```python
from build123d import *

# Parameters (mm, degrees)
SKETCH_1_W          = 10
SKETCH_1_H          = 10
SKETCH_1_W_2        = 8
SKETCH_1_H_2        = 8
EXTRUDE_1_DEPTH     = 20
SKETCH_3_R          = 1.6
CUT_EXTRUDE_1_DEPTH = 23.912878475
SKETCH_4_R          = 1.6
CUT_EXTRUDE_2_DEPTH = 23.912878475


with BuildPart() as part:
    # ｽｹｯﾁ1 → ﾎﾞｽ - 押し出し1 (new body)
    with BuildSketch(Plane.XY):
        Rectangle(SKETCH_1_W, SKETCH_1_H)
        Rectangle(SKETCH_1_W_2, SKETCH_1_H_2, mode=Mode.SUBTRACT)
    extrude(amount=EXTRUDE_1_DEPTH)

    # ｽｹｯﾁ3 → ｶｯﾄ - 押し出し1 (cut, through all)
    with BuildSketch(Plane(origin=(0, 5, 0), x_dir=(1, 0, 0), z_dir=(0, 1, 0))):
        with Locations(Location((0, -5, 0), (0, 0, 270))):
            Circle(SKETCH_3_R)
    extrude(amount=-CUT_EXTRUDE_1_DEPTH, mode=Mode.SUBTRACT)

    # ｽｹｯﾁ4 → ｶｯﾄ - 押し出し2 (cut, through all)
    with BuildSketch(Plane.ZY.offset(5)):
        with Locations(Location((15, 0, 0), (0, 0, 270))):
            Circle(SKETCH_4_R)
    extrude(amount=-CUT_EXTRUDE_2_DEPTH, mode=Mode.SUBTRACT)


solid = part.part
```
The model under review builds one solid part; all positions refer to its coordinate system, in mm. A direction names the side the tool comes from. Round coordinates to 2 decimals unless told otherwise and drop trailing zeros. Loops run counter-clockwise (first coordinate to the right, second up) from the corner with the lowest first, then second, coordinate; pieces in that order, holes last. Notation, with made-up numbers: (-17.75, 76.25) -> (8.25, 76.25) arc R19 ccw to (8.25, 104.25) -> close; hole circle Ø9 at (22.25, 17). An arc over 180 degrees is marked (long way). Answer as a JSON object with one key per item and string values. Group by question number.
1) We need section A-A on x = -3.75. Write out the cut boundary in (y, z), then the cut area to 3 significant figures.
2) For line 1 (X direction, y = 0, z = 2.25); line 2 (X direction, y = 4.25, z = 5.5), list the stretches that pass through material, from the lowest coordinate up. Write a range as [from, to].
3) Mouldability with a two-part tool opening along Y and no side actions: class faces 3 (the face through (5, 0, 10)), 4 (the face through (0, -5, 10)), 5 (the face through (0, 4, 10)) as released by +Y, released by -Y, zero draft, split by the parting line, or undercut.
4) We need section B-B on z = 9.25. Write out the cut boundary in (x, y).
5) We need section C-C on y = 0. Write out the cut boundary in (x, z), then the cut area to 3 significant figures.
6) For pin 1 Ø3.5 at (x, z) = (0, 5) entering from +Y, flat-tipped, find the tip position at first contact; note if it passes through.
7) For faces 1 (the face through (-4.5, 0.1, 0)), 2 (the face through (-4, 0, 10)), list the 3-axis set-ups (+Z, -Z, +X, -X, +Y, -Y) from which the entire face can be reached by the end or side of a thin tool; tool diameter is ignored.
Result set:
{
 "1": {"outline": "(-5, 0) -> (-4, 0) -> (-4, 20) -> (-5, 20) -> close; (4, 0) -> (5, 0) -> (5, 20) -> (4, 20) -> close", "area": "40.0 mm²"},
 "2": {"line 1": "[-5, -4], [4, 5]", "line 2": "[-5, -1.52], [1.52, 5]"},
 "3": {"face 3": "zero draft", "face 4": "released by -Y", "face 5": "undercut"},
 "4": {"outline": "(-5, -5) -> (5, -5) -> (5, 5) -> (-5, 5) -> close; hole (-4, -4) -> (4, -4) -> (4, 4) -> (-4, 4) -> close"},
 "5": {"outline": "(-5, 0) -> (-4, 0) -> (-4, 13.4) -> (-5, 13.4) -> close; (-5, 16.6) -> (-4, 16.6) -> (-4, 20) -> (-5, 20) -> close; (4, 0) -> (5, 0) -> (5, 13.4) -> (4, 13.4) -> close; (4, 16.6) -> (5, 16.6) -> (5, 20) -> (4, 20) -> close", "area": "33.6 mm²"},
 "6": {"pin 1": "y = 5"},
 "7": {"face 1": "-Z, +X, -X, +Y, -Y", "face 2": "+Z, -Z"}
}
